from build123d import *

# Parameters (mm, degrees)
SKETCH1_W                = 177.8
SKETCH1_H                = 101.6
BOSS_EXTRUDE1_DEPTH      = 101.6
CUT_EXTRUDE7_DEPTH       = 1
CUT_EXTRUDE7_DEPTH_BACK  = 76.2
CUT_EXTRUDE10_DEPTH      = 50.8
CUT_EXTRUDE12_DEPTH      = 1
CUT_EXTRUDE12_DEPTH_BACK = 101.6
CUT_EXTRUDE22_DEPTH      = 50.8
CUT_EXTRUDE25_DEPTH      = 50.8


with BuildPart() as part:
    # Sketch1 → Boss-Extrude1 (new body)
    with BuildSketch(Plane(origin=(0, 0, 0), x_dir=(1, 0, 0), z_dir=(0, 1, 0))):
        with Locations((88.9, 50.8)):
            Rectangle(SKETCH1_W, SKETCH1_H)
    extrude(amount=BOSS_EXTRUDE1_DEPTH)

    # Sketch2 → Cut-Extrude7 (cut, two sides)
    with BuildSketch(Plane.ZY) as cut_extrude7_sk:
        Polygon((210.271067812, -159.471067812), (0, 50.8), (-50.8, 101.6), (0, 101.6), (297.368195874, 101.6), (861.537049505, -86.614984162), (774.439921442, -347.686051974), align=None)
    extrude(amount=CUT_EXTRUDE7_DEPTH, mode=Mode.SUBTRACT)
    extrude(cut_extrude7_sk.sketch, amount=-CUT_EXTRUDE7_DEPTH_BACK, mode=Mode.SUBTRACT)

    # Sketch6 → Cut-Extrude10 (cut)
    with BuildSketch(Plane(origin=(0, 0, 0), x_dir=(1, 0, 0), z_dir=(0, 1, 0))):
        Polygon((76.2, 0), (177.8, 50.8), (177.8, 0), align=None)
    extrude(amount=CUT_EXTRUDE10_DEPTH, mode=Mode.SUBTRACT)

    # Sketch8 → Cut-Extrude12 (cut, two sides)
    with BuildSketch(Plane(origin=(0, 101.6, 0), x_dir=(1, 0, 0), z_dir=(0, 1, 0))) as cut_extrude12_sk:
        Polygon((177.8, 50.8), (76.2, 0), (177.8, 0), align=None)
    extrude(amount=CUT_EXTRUDE12_DEPTH, mode=Mode.SUBTRACT)
    extrude(cut_extrude12_sk.sketch, amount=-CUT_EXTRUDE12_DEPTH_BACK, mode=Mode.SUBTRACT)

    # Sketch11 → Cut-Extrude22 (cut)
    with BuildSketch(Plane(origin=(0, 101.6, 0), x_dir=(1, 0, 0), z_dir=(0, 1, 0))):
        Polygon((177.8, 50.8), (76.2, 50.8), (76.2, 0), align=None)
    extrude(amount=-CUT_EXTRUDE22_DEPTH, mode=Mode.SUBTRACT)

    # Sketch15 → Cut-Extrude25 (cut)
    with BuildSketch(Plane.XY.offset(-50.8)):
        Polygon((177.8, 50.8), (76.2, 101.6), (177.8, 101.6), align=None)
    extrude(amount=-CUT_EXTRUDE25_DEPTH, mode=Mode.SUBTRACT)


solid = part.part
Model file for the job. Use its own axes, mm. A direction names the side the tool comes from. Coordinates: 2 decimals unless noted, no trailing zeros. Order: outer loops, then holes, each group sorted by start corner. A loop starts at its lowest first (then second) coordinate and runs counter-clockwise, first axis right, second up. Notation, with made-up numbers: (40, -2.75) -> (48, -2.75) arc R25 ccw to (48, 9.25) -> close; hole circle Ø4 at (29.5, 30). An arc over 180 degrees is marked (long way). Return JSON: item names as keys, results as strings. Group by question number.
Item 1: Saw through at A-A on z = -27. Write the cut outline in (x, y).
Item 2: Flat gauge pins, fed straight in: P1, Ø1, axis at x = 49, z = -20.5, coming from the +Y side; P2, Ø6, axis at x = 43.5, z = -10, coming from the +Y side; P3, Ø1.5, axis at x = 80.5, y = 32.5, coming from the +Z side (3 decimals); P4, Ø15, axis at x = 145, y = 83.5, coming from the +Z side. Where does each tip first touch, or does it go through?
Item 3: Saw through at C-C on y = 9. Write the cut outline in (x, z).
Item 4: Saw through at B-B on x = 137. Write the cut outline in (y, z).
Item 5: Saw through at D-D on x = 37. Write the cut outline in (y, z).
Item 6: Tool access for faces 1 (the flat face through (115, 50.8, -31)), 2 (the flat face through (88, 50, -101.6)): list every direction of +Z, -Z, +X, -X, +Y, -Y with a clear straight run to the whole face (end or side of a thin tool).
Item 7: Wall check: line 1 along Z through (x, y) = (98.5, 64.5); line 2 along Y through (x, z) = (130.5, -41.5); line 3 along X through (y, z) = (87, -40.5). Give the ranges that are in metal, low to high. Write a range as [from, to].
Values found:
{
 "1": {"outline": "(0, 0) -> (130.2, 0) -> (130.2, 50.8) -> (76.2, 50.8) -> (76.2, 77.8) -> (0, 77.8) -> close"},
 "2": {"P1": "stops at y = 71.8", "P2": "stops at y = 63.8", "P3": "stops at z = -1.775", "P4": "passes through"},
 "3": {"outline": "(0, -101.6) -> (177.8, -101.6) -> (177.8, -50.8) -> (76.2, 0) -> (0, 0) -> close"},
 "4": {"outline": "(0, -101.6) -> (71.2, -101.6) -> (71.2, -50.8) -> (50.8, -50.8) -> (50.8, -30.4) -> (0, -30.4) -> close"},
 "5": {"outline": "(0, -101.6) -> (101.6, -101.6) -> (101.6, -50.8) -> (50.8, 0) -> (0, 0) -> close"},
 "6": {"face 1": "+Z, +X, +Y", "face 2": "-Z, +X, -X, +Y, -Y"},
 "7": {"line 1": "z = [-101.6, -50.8]", "line 2": "y = [0, 50.8]", "line 3": "x = [0, 76.2]"}
}
